```python
from build123d import *

# Parameters (mm, degrees)
SKETCH1_R           = 11
BOSS_EXTRUDE1_DEPTH = 7
CUT_EXTRUDE1_DEPTH  = 8
SKETCH5_R           = 2
CUT_EXTRUDE2_DEPTH  = 8


with BuildPart() as part:
    # Sketch1 → Boss-Extrude1 (new body)
    with BuildSketch(Plane.XY):
        with BuildLine():
            Line((42.143593539, 104.994845224), (-13.856406461, 8))
            ThreePointArc((-13.856406461, 8), (-13.856406461, -8), (0, -16))
            Line((0, -16), (112, -16))
            ThreePointArc((112, -16), (125.856406461, -8), (125.856406461, 8))
            Line((125.856406461, 8), (69.856406461, 104.994845224))
            ThreePointArc((69.856406461, 104.994845224), (56, 112.994845224), (42.143593539, 104.994845224))
        make_face()
        Circle(SKETCH1_R, mode=Mode.SUBTRACT)
        with Locations((112, 0)):
            Circle(SKETCH1_R, mode=Mode.SUBTRACT)
        with Locations((56, 96.994845224)):
            Circle(SKETCH1_R, mode=Mode.SUBTRACT)
    extrude(amount=BOSS_EXTRUDE1_DEPTH)

    # Sketch2 → Cut-Extrude1 (cut, through all)
    with BuildSketch(Plane.XY.offset(7)):
        with BuildLine():
            Line((9.622063078, 18.665902125), (23.383974596, 42.502232084))
            Line((23.383974596, 42.502232084), (48.5, 28.001488056))
            Line((48.5, 28.001488056), (48.5, -1))
            Line((48.5, -1), (20.976176963, -1))
            ThreePointArc((20.976176963, -1), (18.186533479, 10.5), (9.622063078, 18.665902125))
        make_face()
        with BuildLine():
            Line((63.5, -1), (91.023823037, -1))
            ThreePointArc((91.023823037, -1), (93.813466521, 10.5), (102.377936922, 18.665902125))
            Line((102.377936922, 18.665902125), (88.616025404, 42.502232084))
            Line((88.616025404, 42.502232084), (63.5, 28.001488056))
            Line((63.5, 28.001488056), (63.5, -1))
        make_face()
        with BuildLine():
            Line((30.883974596, 55.49261314), (44.645886115, 79.328943099))
            ThreePointArc((44.645886115, 79.328943099), (56, 75.994845224), (67.354113885, 79.328943099))
            Line((67.354113885, 79.328943099), (81.116025404, 55.49261314))
            Line((81.116025404, 55.49261314), (56, 40.991869112))
            Line((56, 40.991869112), (30.883974596, 55.49261314))
        make_face()
    extrude(amount=-CUT_EXTRUDE1_DEPTH, mode=Mode.SUBTRACT)

    # Sketch5 → Cut-Extrude2 (cut, through all)
    with BuildSketch(Plane.XY.offset(7)):
        with Locations((24.388784068, 59.24261314)):
            Circle(SKETCH5_R)
        with Locations((16.888784068, 46.252232084)):
            Circle(SKETCH5_R)
        with Locations((87.611215932, 59.24261314)):
            Circle(SKETCH5_R)
        with Locations((95.111215932, 46.252232084)):
            Circle(SKETCH5_R)
    extrude(amount=-CUT_EXTRUDE2_DEPTH, mode=Mode.SUBTRACT)


solid = part.part
```
Input: part model. Units: mm. Frame: model coordinates. A direction names the side the tool comes from. Coordinates: 2 decimals unless noted, no trailing zeros. Loops run counter-clockwise (first coordinate to the right, second up) from the corner with the lowest first, then second, coordinate; pieces in that order, holes last.
Q1. Mould query, pull axis X, two halves, no side actions, for faces 3 (the flat face through (35.77, 35.35, 3.55)), 4 (the flat face through (14.536, 57.176, 3.451)), 5 (the flat face through (37.669, 67.244, 3.549)), 6 (the flat face through (98.248, 55.818, 3.451)). Classes: +X half, -X half, draft (parallel to the pull), parting line (faces both ways), or undercut.
Results are:
face 3: undercut
face 4: -X half
face 5: undercut
face 6: +X half
Q2. Section D-D, the plane x = 7. Return the cut outline in (y, z).
Results are:
outline: (-16, 0) - (-8.49, 0) - (-8.49, 7) - (-16, 7) - close; (8.49, 0) - (44.12, 0) - (44.12, 7) - (8.49, 7) - close
Q3. Section A-A, the plane x = 34.5. Return the cut outline in (y, z), and give its area (3 significant figures).
Results are:
outline: (-16, 0) - (-1, 0) - (-1, 7) - (-16, 7) - close; (36.08, 0) - (53.4, 0) - (53.4, 7) - (36.08, 7) - close; (61.76, 0) - (91.76, 0) - (91.76, 7) - (61.76, 7) - close
area: 436 mm2
Q4. Section C-C, the plane y = 53. Return the cut outline in (x, z).
Results are:
outline: (12.12, 0) - (35.2, 0) - (35.2, 7) - (12.12, 7) - close; (76.8, 0) - (99.88, 0) - (99.88, 7) - (76.8, 7) - close
Q5. Set-up query: faces 1 (the cylindrical face through (55.832, 75.996, 3.549)), 2 (the cylindrical face through (125.74, -8.2, 3.45)). Return all of +Z, -Z, +X, -X, +Y, -Y with unobstructed straight access to the full face (end or side cutting, diameter ignored); none if empty.
Results are:
face 1: +Z, -Z
face 2: +Z, -Z, +X
Q6. Line query: line 1 along X through (y, z) = (36.5, 5); line 2 along Y through (x, z) = (55, 5.75); line 3 along X through (y, z) = (9.5, 5.75). Output: solid intervals per line, ascending.
Results are:
line 1: x = 2.6 to 19.92, 33.78 to 78.22, 92.08 to 109.4
line 2: y = -16 to 41.57, 76.02 to 86.04, 107.95 to 112.96
line 3: x = -12.99 to -5.55, 5.55 to 18.73, 48.5 to 63.5, 93.27 to 106.45, 117.55 to 124.99
Q7. Section B-B, the plane z = 4.25. Give the number of separate pieces and of enclosed holes in the cut face, and give its area (3 significant figures).
Results are:
separate pieces: 1
enclosed holes: 10
area: 6,870 mm2
Q8. Contact query for flat-ended pins moving along their axis: pin 1 (20 mm diameter, centred on x = 56, y = 96.99, fed in from -Z); pin 2 (2 mm diameter, centred on y = 9.5, z = 3.5, fed in from +X); pin 3 (3.5 mm diameter, centred on x = 32.5, z = 2, fed in from +Y). Output: stop coordinate, or through.
Results are:
pin 1: passes through
pin 2: stops at x = 125.57
pin 3: stops at y = 91.32
